Check sheet for the modelled part. Datum: model origin and axes. Units: mm. Face numbers are marked on the shaded views. A direction names the side the tool comes from. Round coordinates to 2 decimals unless told otherwise and drop trailing zeros. Loops run counter-clockwise (first coordinate to the right, second up) from the corner with the lowest first, then second, coordinate; pieces in that order, holes last. Notation, with made-up numbers: M -12,76.25 L 28,76.25 A15 ccw 28,104.25 Z; hole C 33,49.5 d8. An arc over 180 degrees is marked long. One line per question, with ' | ' between items. Start each with the question number.
(1) Section check D-D (z = 3). Record the boundary of the cut face in (x, y).
(2) Go/stop test with flat-tipped pins: P1, Ø1.5, axis at y = -43, z = 4, coming from the +X side; P2, Ø4, axis at x = -19, y = -15, coming from the -Z side; P3, Ø1.8, axis at x = 16.5, z = 6.5, coming from the -Y side; P4, Ø3, axis at x = 22.5, z = 2, coming from the -Y side. Record where each tip stops, or that it passes through.
(3) Thickness scan on probe 1 along X at (y, z) = (-15, 2.95); probe 2 along Y at (x, z) = (5, 1.55); probe 3 along X at (y, z) = (-11, 5.5) (3 decimals). Record the ranges inside material, lowest first. Write a range as [from, to].
(4) Section check C-C (y = -15). Record the boundary of the cut face in (x, z), and give its area (3 significant figures).
(5) Section check A-A (x = 5). Record the boundary of the cut face in (y, z), and give its area (3 significant figures).
(6) Tool access check on the marked faces 1, 2 and 3. Record the directions out of +Z, -Z, +X, -X, +Y, -Y that give a thin tool (end or side, any length) a straight path to the whole face; none if there is none.
(7) Section check B-B (z = 7). Record the boundary of the cut face in (x, y) (3 decimals).
```python
from build123d import *

# Parameters (mm, degrees)
F0_R     = 1.65
F1_DEPTH = 4
F2_W     = 10
F2_H     = 2.5
F3_DEPTH = 6
F4_R     = 1.65
F5_DEPTH = 12.501


with BuildPart() as f1:
    # F0 (on Top) → F1 (new body)
    with BuildSketch(Plane.XY):
        Polygon((10, 0), (0, 0), (0, -10), (-24, -10), (-24, -20), (0, -20), (0, -50), (10, -50), (10, -20), (34, -20), (34, -10), (10, -10), align=None)
        with Locations((-19, -15)):
            Circle(F0_R, mode=Mode.SUBTRACT)
        with Locations((29, -15)):
            Circle(F0_R, mode=Mode.SUBTRACT)
        with Locations((5, -5.4125)):
            Circle(F0_R, mode=Mode.SUBTRACT)
    extrude(amount=F1_DEPTH)

    # F2 (on face) → F3 (join)
    with BuildSketch(Plane.XY.offset(4)):
        with Locations((-8.675, -11.25)):
            Rectangle(F2_W, F2_H)
    extrude(amount=F3_DEPTH)

    # F4 (on face) → F5 (cut, through all)
    with BuildSketch(Plane.XZ.offset(12.5)):
        with Locations((-8.675, 7)):
            Circle(F4_R)
    extrude(amount=-F5_DEPTH, mode=Mode.SUBTRACT)

    # F7: F1 across plane


with BuildPart() as f1_1:
    add(f1.part)
    add(f1.part.mirror(Plane(origin=(5, -35, 2), x_dir=(0, 1, 0), z_dir=(1, 0, 0))))


solid = f1_1.part
```
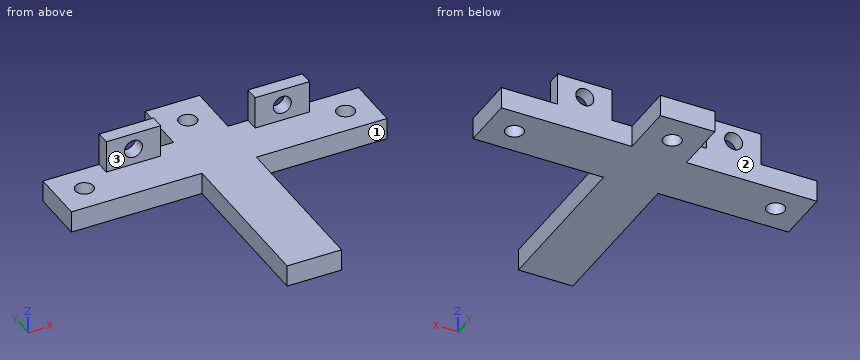
The answers:
1) outline: M -24,-20 L 0,-20 L 0,-50 L 10,-50 L 10,-20 L 34,-20 L 34,-10 L 10,-10 L 10,0 L 0,0 L 0,-10 L -24,-10 Z; hole C -19,-15 d3.3; hole C 5,-5.41 d3.3; hole C 29,-15 d3.3
2) P1: x = 10 | P2: z = 0 | P3: y = -12.5 | P4: y = -20
3) probe 1: [-24, -20.65], [-17.35, 27.35], [30.65, 34] | probe 2: [-50, -7.06], [-3.76, 0] | probe 3: [-13.675, -9.362], [-7.988, -3.675], [13.675, 17.988], [19.362, 23.675]
4) outline: M -24,0 L -20.65,0 L -20.65,4 L -24,4 Z; M -17.35,0 L 27.35,0 L 27.35,4 L -17.35,4 Z; M 30.65,0 L 34,0 L 34,4 L 30.65,4 Z | area: 206 mm²
5) outline: M -50,0 L -7.06,0 L -7.06,4 L -50,4 Z; M -3.76,0 L 0,0 L 0,4 L -3.76,4 Z | area: 187 mm²
6) face 1: +Z, -Z, +X, -Y | face 2: +Z, -Z, -X, +Y | face 3: +Z, +X, -X, -Y
7) outline: M -13.675,-12.5 L -10.325,-12.5 L -10.325,-10 L -13.675,-10 Z; M -7.025,-12.5 L -3.675,-12.5 L -3.675,-10 L -7.025,-10 Z; M 13.675,-12.5 L 17.025,-12.5 L 17.025,-10 L 13.675,-10 Z; M 20.325,-12.5 L 23.675,-12.5 L 23.675,-10 L 20.325,-10 Z
